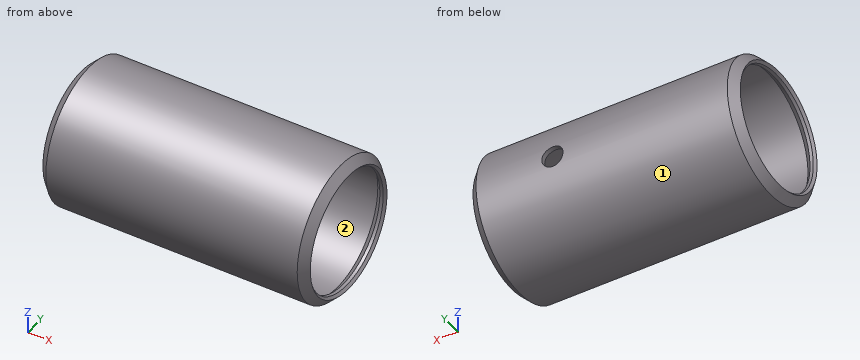
Autodesk Inventor part; units mm, degrees
ref_plane "o1_XY" through (0, -7.8105, 0) normal (1, 0, 0) x (0, 0, -1)
ref_plane "o1_YZ" through (0, -7.8105, 0) normal (0, 0, -1) x (0, 1, 0)
ref_plane "o1_ZX" through (0, -7.8105, 0) normal (0, 1, 0) x (1, 0, 0)
sketch "Sketch_5" plane through (0, 0, 0) normal (0, 0, 1) x (1, 0, 0)
  line L0 (30.1752, 0) -> (-30.1752, 0)
  line L1 (0, 6.9051) -> (0.263, 6.6421)
  line L2 (0.263, 6.6421) -> (0.635, 6.6421)
  line L3 (0.635, 6.6421) -> (1.27, 7.2771)
  line L4 (1.27, 7.2771) -> (28.9052, 7.2771)
  line L5 (28.9052, 7.2771) -> (29.5402, 6.6421)
  line L6 (29.5402, 6.6421) -> (29.9122, 6.6421)
  line L7 (29.9122, 6.6421) -> (30.1752, 6.9051)
  line L8 (30.1752, 6.9051) -> (29.2698, 7.8105)
  line L9 (29.2698, 7.8105) -> (0.9054, 7.8105)
  line L10 (0.9054, 7.8105) -> (0, 6.9051)
revolve "Revolution1" add sketch "Sketch_5" angle 360 about axis through (30.1752, 0, 0) along (1, 0, 0)
sketch "Sketch_1" plane through (0, 0, 0) normal (0, 0, 1) x (1, 0, 0)
  line L0 (20.6502, 0) -> (20.6502, 7.8105)
  line L1 (20.6502, 7.8105) -> (21.844, 7.8105)
  line L2 (21.844, 7.8105) -> (21.844, 0)
  line L3 (21.844, 0) -> (20.6502, 0)
  line L4 (20.6502, 0) -> (20.6502, 7.8105)
revolve "Revolution2" cut sketch "Sketch_1" angle 360 about axis through (20.6502, 0, 0) along (0, -1, 0)
ref_plane "o1_XY" through (0, -7.8105, 0) normal (1, 0, 0) x (0, 0, -1)
ref_plane "o1_YZ" through (0, -7.8105, 0) normal (0, 0, -1) x (0, 1, 0)
ref_plane "o1_ZX" through (0, -7.8105, 0) normal (0, 1, 0) x (1, 0, 0)
ref_plane "o2_XY" through (0, 7.8105, 0) normal (1, 0, 0) x (0, 0, -1)
ref_plane "o2_YZ" through (0, 7.8105, 0) normal (0, 0, -1) x (0, 1, 0)
ref_plane "o2_ZX" through (0, 7.8105, 0) normal (0, 1, 0) x (1, 0, 0)
ref_plane "t1_XY" through (15.0876, 7.8105, 0) normal (1, 0, 0) x (0, 0, -1)
ref_plane "t1_YZ" through (15.0876, 7.8105, 0) normal (0, 0, -1) x (0, 1, 0)
ref_plane "t1_ZX" through (15.0876, 7.8105, 0) normal (0, 1, 0) x (1, 0, 0)
ref_plane "t2_XY" through (15.0876, 0, -7.8105) normal (1, 0, 0) x (0, 0, -1)
ref_plane "t2_YZ" through (15.0876, 0, -7.8105) normal (0, 0, -1) x (0, 1, 0)
ref_plane "t2_ZX" through (15.0876, 0, -7.8105) normal (0, 1, 0) x (1, 0, 0)
ref_plane "t3_XY" through (15.0876, -7.8105, 0) normal (1, 0, 0) x (0, 0, -1)
ref_plane "t3_YZ" through (15.0876, -7.8105, 0) normal (0, 0, -1) x (0, 1, 0)
ref_plane "t3_ZX" through (15.0876, -7.8105, 0) normal (0, 1, 0) x (1, 0, 0)
ref_plane "t4_XY" through (15.0876, 0, 7.8105) normal (1, 0, 0) x (0, 0, -1)
ref_plane "t4_YZ" through (15.0876, 0, 7.8105) normal (0, 0, -1) x (0, 1, 0)
ref_plane "t4_ZX" through (15.0876, 0, 7.8105) normal (0, 1, 0) x (1, 0, 0)
ref_plane "tube1_XY" through (1.27, 0, 0) normal (1, 0, 0) x (0, 0, -1)
ref_plane "tube1_YZ" through (1.27, 0, 0) normal (0, 0, -1) x (0, 1, 0)
ref_plane "tube1_ZX" through (1.27, 0, 0) normal (0, 1, 0) x (1, 0, 0)
ref_plane "tube2_XY" through (28.9052, 0, 0) normal (1, 0, 0) x (0, 0, -1)
ref_plane "tube2_YZ" through (28.9052, 0, 0) normal (0, 0, -1) x (0, 1, 0)
ref_plane "tube2_ZX" through (28.9052, 0, 0) normal (0, 1, 0) x (1, 0, 0)
properties part number "D-75938XP-1.188"
Here's how the part is built. I have some questions about the finished solid (model axes, mm). Face numbers are marked on the shaded views. Coordinates: 2 decimals unless noted, no trailing zeros. Loops run counter-clockwise (first coordinate to the right, second up) from the corner with the lowest first, then second, coordinate; pieces in that order, holes last. Notation, with made-up numbers: (50, 74) -> (72, 74) arc R12 cw to (72, 80) -> close; hole circle Ø5 at (27, 26). An arc over 180 degrees is marked (long way). Use one line per item in the form item = value. Start each with the question number.
(1) If we section it at D-D (x = 21): Please give me the cut outline in (y, z), then the cut area to 3 significant figures.
(2) We'd pull the mould along Z, two halves only. Please class the marked faces 1 and 2: pulls with the +Z half, pulls with the -Z half, needs draft (parallel to the pull), parting line crosses it, or undercut.
(3) Please list where these lines run through material, in increasing order: line 1 along X through (y, z) = (7.55, 0); line 2 along Y through (x, z) = (3.5, 2.5); line 3 along Z through (x, y) = (16.5, -2).
(4) If we section it at C-C (x = 4.5): Please give me the cut outline in (y, z).
(5) If we section it at A-A (z = 0): Give the number of separate pieces and of enclosed holes in the cut face, then the cut area to 3 significant figures.
(6) Will these pins go through, and if not, where does the flat tip stop? pin 1 (8 mm diameter, centred on x = 17, z = 3, fed in from -Y); pin 2 (1 mm diameter, centred on x = 5.5, y = 1, fed in from +Z); pin 3 (4 mm diameter, centred on y = 1.5, z = -4.5, fed in from +X); pin 4 (5 mm diameter, centred on x = 5, y = -4.5, fed in from +Z).
Verdict:
q1.outline = (7.19, -1.14) arc R7.28 cw (long way) to (7.19, 1.14) -> (7.73, 1.14) arc R7.81 ccw (long way) to (7.73, -1.14) -> close
q1.area = 24.1 mm²
q2.face_1 = parting line crosses it
q2.face_2 = undercut
q3.line_1 = 0.64 to 19.46, 21.84 to 29.53
q3.line_2 = -7.4 to -6.83, 6.83 to 7.4
q3.line_3 = -7.55 to -7, 7 to 7.55
q4.outline = circle Ø15.62 at (0, 0); hole circle Ø14.55 at (0, 0)
q5.separate_pieces = 3
q5.enclosed_holes = 0
q5.area = 31.6 mm²
q6.pin_1 = -7.81
q6.pin_2 = 7.79
q6.pin_3 = 30.01
q6.pin_4 = 7.55
